from build123d import *

# Parameters (mm, degrees)
BOSS_EXTRUDE1_DEPTH     = 20
FILLET1_R               = 4
SKETCH2_R               = 2.75
CUT_EXTRUDE1_DEPTH      = 1.5
LPATTERN1_COUNT         = 3
LPATTERN1_PITCH         = 30
CUT_EXTRUDE2_DEPTH      = 48.236109069
CUT_EXTRUDE2_DEPTH_BACK = 48.236109069
WRAP1_DEPTH             = 1


# Read off the part's stored shape, not the designer's step: Wrap1
with BuildPart() as part:
    # Sketch1 → Boss-Extrude1 (new body)
    with BuildSketch(Plane(origin=(0, 0, 0), x_dir=(1, 0, 0), z_dir=(0, 1, 0))):
        with BuildLine():
            Line((37.5, -5), (-37.5, -5))
            ThreePointArc((-37.5, -5), (-42.5, 0), (-37.5, 5))
            Line((-37.5, 5), (37.5, 5))
            ThreePointArc((37.5, 5), (42.5, 0), (37.5, -5))
        make_face()
    extrude(amount=BOSS_EXTRUDE1_DEPTH)

    # Fillet1
    fillet1_edges = [part.edges().sort_by_distance(p)[0] for p in [
        (-42.5, 20, 0),
        (0, 20, 5),
        (42.5, 20, 0),
        (0, 20, -5),
    ]]
    fillet(fillet1_edges, radius=FILLET1_R)

    # Sketch2 → Cut-Extrude1 (cut)
    with BuildSketch(Plane.XZ):
        with Locations(Location((-37.5, 0, 0), (0, 0, 270))):
            Circle(SKETCH2_R)
    cut_extrude1 = extrude(amount=-CUT_EXTRUDE1_DEPTH, mode=Mode.SUBTRACT)

    # LPattern1: Cut-Extrude1 ×3
    with Locations(*[(i * LPATTERN1_PITCH, 0, 0) for i in range(1, LPATTERN1_COUNT)]):
        add(cut_extrude1, mode=Mode.SUBTRACT)

    # Sketch3 → Cut-Extrude2 (cut, two sides: drawn at the far end of the back side and taken through both)
    with BuildSketch(Plane.XY.offset(-CUT_EXTRUDE2_DEPTH_BACK)):
        with BuildLine():
            Line((-5, 23), (5, 23))
            ThreePointArc((5, 23), (8, 20), (5, 17))
            Line((5, 17), (-5, 17))
            ThreePointArc((-5, 17), (-8, 20), (-5, 23))
        make_face()
    extrude(amount=CUT_EXTRUDE2_DEPTH + CUT_EXTRUDE2_DEPTH_BACK, mode=Mode.SUBTRACT)

    # Wrap1 outline → Wrap1 (add)
    with BuildSketch(Plane(origin=(0, 17, 0), x_dir=(1, 0, 0), z_dir=(0, 1, 0))):
        with BuildLine():
            add(Edge.make_bspline(
                [(1.477179672, -2.131048558), (1.531961531, -2.129025799), (1.636756934, -2.125156347), (1.784042683, -2.083710764), (1.912739128, -2.017798162), (2.002734413, -1.937441096), (2.063880351, -1.856422731), (2.108803156, -1.780024303), (2.151677105, -1.688112446), (2.192727948, -1.580807318), (2.232736726, -1.458316815), (2.27140835, -1.320528166), (2.305449427, -1.166588854), (2.327738483, -1.058958074), (2.339359159, -1.00284343)],
                knots=[0, 0, 0, 0, 0.10403341, 0.199011557, 0.288612319, 0.377191825, 0.425797175, 0.481425289, 0.545557079, 0.61863331, 0.699984683, 0.790771883, 0.890916323, 1, 1, 1, 1], degree=3))
            Line((1.477179672, -2.131048558), (-0.993974174, -2.131048558))
            add(Edge.make_bspline(
                [(0.868205313, -0.597394712), (0.79621048, -0.649910777), (0.657741061, -0.750916207), (0.456580944, -0.893601927), (0.27646951, -1.029215281), (0.111636193, -1.150958881), (-0.034458066, -1.262447791), (-0.163409095, -1.362077669), (-0.274143139, -1.450060052), (-0.45325139, -1.598443158), (-0.698599089, -1.817172559), (-0.896074552, -2.027016962), (-0.993974174, -2.131048558)],
                knots=[0, 0, 0, 0, 0.110593572, 0.212707314, 0.306051588, 0.390379305, 0.467018215, 0.534117187, 0.592614819, 0.642525788, 0.822780058, 1, 1, 1, 1], degree=3))
            add(Edge.make_bspline(
                [(2.611795057, 1.311259134), (2.575402231, 1.227702286), (2.503450629, 1.062503542), (2.369097378, 0.829017261), (2.221591228, 0.607376082), (2.079695352, 0.434265273), (1.953675403, 0.296924311), (1.842689454, 0.188702281), (1.717579256, 0.073349805), (1.577787564, -0.048748331), (1.422213899, -0.176924213), (1.250181802, -0.310729341), (1.06539278, -0.453791096), (0.935229638, -0.548583621), (0.868205313, -0.597394712)],
                knots=[0, 0, 0, 0, 0.10413489, 0.205883221, 0.307528832, 0.408265615, 0.461433854, 0.520606469, 0.585444086, 0.656004792, 0.732803839, 0.815893726, 0.905198979, 1, 1, 1, 1], degree=3))
            add(Edge.make_bspline(
                [(2.767243775, 2.136579647), (2.765476042, 2.062762359), (2.762016076, 1.918280503), (2.73244702, 1.70614551), (2.6833885, 1.503661888), (2.635496742, 1.374955883), (2.611795057, 1.311259134)],
                knots=[0, 0, 0, 0, 0.261979501, 0.512769921, 0.758869279, 1, 1, 1, 1], degree=3))
            add(Edge.make_bspline(
                [(0.446730954, 4.125361698), (0.531185697, 4.123275975), (0.696746898, 4.119187219), (0.939241519, 4.094203646), (1.169092432, 4.04891417), (1.386926246, 3.987244257), (1.590639541, 3.904356397), (1.783380165, 3.807151368), (1.961901465, 3.688660444), (2.12755051, 3.554901637), (2.277544806, 3.408600033), (2.408670906, 3.251890691), (2.519920579, 3.086706843), (2.609878279, 2.912173499), (2.68146261, 2.730376132), (2.730374873, 2.539782347), (2.762493821, 2.341195944), (2.765641094, 2.205619187), (2.767243775, 2.136579647)],
                knots=[0, 0, 0, 0, 0.074102612, 0.14526736, 0.21355926, 0.279416432, 0.343556942, 0.406228654, 0.468492489, 0.531146675, 0.592790073, 0.652016559, 0.710119813, 0.767135501, 0.823967905, 0.881147087, 0.939476717, 1, 1, 1, 1], degree=3))
            add(Edge.make_bspline(
                [(-1.397820328, 3.42664375), (-1.339685121, 3.482468658), (-1.223933781, 3.593620027), (-1.029988725, 3.73621049), (-0.821845174, 3.857829356), (-0.597170186, 3.955349696), (-0.357859278, 4.032519936), (-0.102825371, 4.086723136), (0.167059066, 4.118844208), (0.3520908, 4.123156198), (0.446730954, 4.125361698)],
                knots=[0, 0, 0, 0, 0.119107626, 0.23715177, 0.355050392, 0.47498588, 0.598670295, 0.726365388, 0.860041186, 1, 1, 1, 1], degree=3))
            add(Edge.make_bspline(
                [(-1.950704943, 2.013182211), (-1.949501261, 2.082193438), (-1.947130604, 2.218111311), (-1.918428152, 2.417004203), (-1.875210504, 2.607330065), (-1.816463805, 2.790033991), (-1.737178724, 2.962937631), (-1.641872629, 3.127763446), (-1.530076028, 3.284407224), (-1.442173454, 3.378943465), (-1.397820328, 3.42664375)],
                knots=[0, 0, 0, 0, 0.132803649, 0.26155729, 0.386082589, 0.508400008, 0.630401232, 0.751619273, 0.874674186, 1, 1, 1, 1], degree=3))
            add(Edge.make_bspline(
                [(-1.011602379, 0.740746314), (-1.076799531, 0.74447446), (-1.204521956, 0.751777966), (-1.386461074, 0.818290605), (-1.550070508, 0.925271117), (-1.69322001, 1.073400563), (-1.811500845, 1.259061279), (-1.890938186, 1.482580071), (-1.943991337, 1.736660149), (-1.9483889, 1.917788326), (-1.950704943, 2.013182211)],
                knots=[0, 0, 0, 0, 0.110139331, 0.215764983, 0.323707128, 0.438906263, 0.562183724, 0.693638164, 0.838649921, 1, 1, 1, 1], degree=3))
            add(Edge.make_bspline(
                [(-0.104551097, 1.612541186), (-0.107433277, 1.55184237), (-0.113041089, 1.433741609), (-0.162702617, 1.264530911), (-0.246008733, 1.112720856), (-0.36059696, 0.981658482), (-0.497861102, 0.874736466), (-0.653954588, 0.794785259), (-0.828098239, 0.750308211), (-0.94939653, 0.74398769), (-1.011602379, 0.740746314)],
                knots=[0, 0, 0, 0, 0.129242333, 0.251464839, 0.372304265, 0.495878621, 0.620081591, 0.741344555, 0.867352775, 1, 1, 1, 1], degree=3))
            add(Edge.make_bspline(
                [(-0.764807507, 2.352925801), (-0.712490789, 2.337787093), (-0.613060164, 2.309015197), (-0.477694691, 2.245410486), (-0.363497683, 2.17010385), (-0.266944344, 2.084386734), (-0.194142589, 1.983320843), (-0.142356861, 1.870047676), (-0.108753882, 1.745331032), (-0.105978345, 1.657636068), (-0.104551097, 1.612541186)],
                knots=[0, 0, 0, 0, 0.151156851, 0.287281401, 0.413669873, 0.530293514, 0.644009236, 0.756908248, 0.874996313, 1, 1, 1, 1], degree=3))
            add(Edge.make_bspline(
                [(-1.151025456, 2.508374519), (-1.133287913, 2.494836068), (-1.091141008, 2.462666798), (-1.005178361, 2.42780874), (-0.895290257, 2.386647547), (-0.811045884, 2.364875571), (-0.764807507, 2.352925801)],
                knots=[0, 0, 0, 0, 0.159109439, 0.378066483, 0.65864549, 1, 1, 1, 1], degree=3))
            add(Edge.make_bspline(
                [(-1.232756225, 2.707092468), (-1.232081899, 2.687184305), (-1.230781196, 2.648783562), (-1.21372537, 2.594957911), (-1.188222188, 2.546850656), (-1.163446829, 2.521223132), (-1.151025456, 2.508374519)],
                knots=[0, 0, 0, 0, 0.268945253, 0.518766978, 0.758729042, 1, 1, 1, 1], degree=3))
            add(Edge.make_bspline(
                [(-0.00038443, 3.612541186), (-0.085081224, 3.608833937), (-0.24886475, 3.601664997), (-0.483889311, 3.546755047), (-0.696299395, 3.452253769), (-0.880349687, 3.323453619), (-1.031886602, 3.177298589), (-1.146772165, 3.025778423), (-1.218404743, 2.867863556), (-1.228074056, 2.759544014), (-1.232756225, 2.707092468)],
                knots=[0, 0, 0, 0, 0.151816317, 0.293576777, 0.429964406, 0.566304914, 0.694365033, 0.806085808, 0.906100976, 1, 1, 1, 1], degree=3))
            add(Edge.make_bspline(
                [(1.126218134, 2.202284775), (1.125419382, 2.258418172), (1.123872297, 2.367141747), (1.108484739, 2.524352927), (1.087625139, 2.671598252), (1.052679442, 2.807704167), (1.012774581, 2.935365364), (0.958393781, 3.050865278), (0.898520263, 3.157786792), (0.826714952, 3.252443042), (0.749134805, 3.338292119), (0.661001364, 3.410228111), (0.568127793, 3.473318886), (0.468377407, 3.525349279), (0.360714304, 3.563257103), (0.247252366, 3.592895766), (0.125557638, 3.608210727), (0.042385847, 3.61107055), (-0.00038443, 3.612541186)],
                knots=[0, 0, 0, 0, 0.082284271, 0.159374645, 0.231497254, 0.300083139, 0.36523236, 0.427274673, 0.486932074, 0.544586116, 0.60112786, 0.656190593, 0.710940404, 0.765594865, 0.820607428, 0.877984079, 0.93725451, 1, 1, 1, 1], degree=3))
            add(Edge.make_bspline(
                [(0.714359159, 0.617348878), (0.747261882, 0.682124329), (0.812482722, 0.810524323), (0.894486195, 1.008253415), (0.968284969, 1.205271239), (1.025200713, 1.404323571), (1.07052621, 1.603312874), (1.102444977, 1.802435759), (1.122559216, 2.002082393), (1.124996917, 2.135464326), (1.126218134, 2.202284775)],
                knots=[0, 0, 0, 0, 0.131745637, 0.261150462, 0.388067803, 0.513189353, 0.636374668, 0.758087597, 0.878808958, 1, 1, 1, 1], degree=3))
            add(Edge.make_bspline(
                [(-0.607756225, -1.126240866), (-0.526341272, -1.032411706), (-0.369395008, -0.851534171), (-0.147005377, -0.58818052), (0.052485983, -0.342553042), (0.228461917, -0.115210972), (0.383373607, 0.093014827), (0.514393948, 0.283577403), (0.625301777, 0.454674177), (0.686096112, 0.565722807), (0.714359159, 0.617348878)],
                knots=[0, 0, 0, 0, 0.170005554, 0.327725258, 0.471696803, 0.603008639, 0.721148947, 0.826797124, 0.919478664, 1, 1, 1, 1], degree=3))
            add(Edge.make_bspline(
                [(-2.155833148, -3.076561379), (-2.120077921, -3.019555215), (-2.042967512, -2.896614628), (-1.906171622, -2.707469654), (-1.750693337, -2.493359905), (-1.565930664, -2.262250728), (-1.361697851, -2.006814917), (-1.131972057, -1.731572481), (-0.87885055, -1.434992601), (-0.700428862, -1.231786555), (-0.607756225, -1.126240866)],
                knots=[0, 0, 0, 0, 0.080973991, 0.174630064, 0.280853316, 0.39944862, 0.530692677, 0.674513651, 0.830941638, 1, 1, 1, 1], degree=3))
            Line((-2.155833148, -3.076561379), (-2.155833148, -3.566945994))
            Line((-2.155833148, -3.566945994), (2.664679672, -3.566945994))
            Line((2.664679672, -3.566945994), (2.869807877, -1.00284343))
            Line((2.869807877, -1.00284343), (2.339359159, -1.00284343))
        make_face()
    extrude(amount=WRAP1_DEPTH)


solid = part.part
Could you check a few things on this model? Use its own coordinates, in mm. A direction names the side the tool comes from. Coordinates: 2 decimals unless noted, no trailing zeros. Order: outer loops, then holes, each group sorted by start corner. A loop starts at its lowest first (then second) coordinate and runs counter-clockwise, first axis right, second up. Notation, with made-up numbers: (-30.75, 17.5) - (4.25, 17.5) arc R17 ccw to (4.25, 36.5) - close; hole circle Ø7 at (42, -20). An arc over 180 degrees is marked (long way). Answer in a Markdown table with one row per item. Add a question column.
(1) If we section it at A-A, the plane x = 22.5: Please give me the cut outline in (y, z).
(2) If we mould it in two halves opening along Z, with no side actions, what happens to faces 1 (the face through (1, 0, 0)), 2 (the face through (-7, 1.5, 0)), 3 (the face through (-42.5, 7.9, 0.1))? For each: released by +Z, released by -Z, zero draft, split by the parting line, or undercut.
(3) If we section it at C-C, the plane x = 14: Please give me the cut outline in (y, z), then the cut area to 3 significant figures.
(4) Will these pins go through, and if not, where does the flat tip stop? pin 1 (3.5 mm diameter, centred on x = -37.5, z = 0, fed in from -Y); pin 2 (3 mm diameter, centred on x = 0, z = -1, fed in from +Y); pin 3 (4 mm diameter, centred on y = 9, z = -3.5, fed in from +X).
(5) If we section it at B-B, the plane y = 8: Please give me the cut outline in (x, z).
(6) On a 3-axis mill with a long thin cutter (end or side, diameter ignored), from which of +Z, -Z, +X, -X, +Y, -Y can I reach the whole of each face in a straight line? I mean faces 4 (the face through (0, 18, 1)), 5 (the face through (-10.185, 0.74, 0.596)), 6 (the face through (-23, 20, 0)). Say none if no direction works.
(7) I need wall thicknesses on L1, parallel to X at y = 1.1, z = 0; L2, parallel to X at y = 5.75, z = 1.25; L3, parallel to Y at x = -12.5, z = 3.25. Which ranges of each line are inside material? Lowest first, please.
Results are:
| question | item | result |
|---|---|---|
| 1 | outline | (0, -5) - (16, -5) arc R4 ccw to (20, -1) - (20, 1) arc R4 ccw to (16, 5) - (0, 5) - (0, 2.75) - (1.5, 2.75) - (1.5, -2.75) - (0, -2.75) - close |
| 2 | face 1 | zero draft |
| 2 | face 2 | undercut |
| 2 | face 3 | split by the parting line |
| 3 | outline | (0, -5) - (16, -5) arc R4 ccw to (20, -1) - (20, 1) arc R4 ccw to (16, 5) - (0, 5) - close |
| 3 | area | 193 mm2 |
| 4 | pin 1 | stops at y = 1.5 |
| 4 | pin 2 | stops at y = 18 |
| 4 | pin 3 | stops at x = 42.27 |
| 5 | outline | (-37.5, -5) - (37.5, -5) arc R5 ccw to (37.5, 5) - (-37.5, 5) arc R5 ccw to start |
| 6 | face 4 | +Z, -Z, +Y |
| 6 | face 5 | -Y |
| 6 | face 6 | +Z, -Z, +X, -X, +Y |
| 7 | L1 | x = -42.5 to -40.25, -34.75 to -10.25, -4.75 to 19.75, 25.25 to 42.5 |
| 7 | L2 | x = -42.34 to 42.34 |
| 7 | L3 | y = 0 to 19.31 |
